Geometry: final body of the model. Coordinates: model frame, mm. A direction names the side the tool comes from. Give positions to 0.01 mm unless a question says otherwise; leave off trailing zeros. Write each loop counter-clockwise with the first axis right and the second up, starting at its lowest first coordinate (ties: lowest second). Pieces come first, ordered by that corner, then holes. Notation, with made-up numbers: (40, 41.25) -> (44, 41.25) arc R25 ccw to (44, 67.25) -> close; hole circle Ø3 at (-0.75, 44.5). An arc over 180 degrees is marked (long way). Answer as a JSON object with one key per item and string values.
from build123d import *

# Parameters (mm, degrees)
F1_DEPTH = 25


with BuildPart() as f1:
    # F0 (on Top) → F1 (new body)
    with BuildSketch(Plane.XY):
        with BuildLine():
            ThreePointArc((-17.217742, 262.83602), (-229.349777, 174.968054), (-317.217742, -37.16398))
            Line((-317.217742, -37.16398), (-287.217742, -37.16398))
            ThreePointArc((-287.217742, -37.16398), (-286.799458, -22.140706), (-285.5459, -7.16398))
            ThreePointArc((-285.5459, -7.16398), (-256.973949, 87.001077), (-196.554829, 164.673106))
            ThreePointArc((-196.554829, 164.673106), (-190.879041, 169.576808), (-185.069229, 174.320956))
            ThreePointArc((-185.069229, 174.320956), (-109.629828, 216.52876), (-24.717742, 232.731833))
            ThreePointArc((-24.717742, 232.731833), (-17.217742, 232.83602), (-9.717742, 232.731833))
            ThreePointArc((-9.717742, 232.731833), (75.194344, 216.52876), (150.633745, 174.320956))
            ThreePointArc((150.633745, 174.320956), (156.443556, 169.576808), (162.119344, 164.673106))
            ThreePointArc((162.119344, 164.673106), (222.538464, 87.001077), (251.110415, -7.16398))
            ThreePointArc((251.110415, -7.16398), (252.363973, -22.140706), (252.782258, -37.16398))
            Line((252.782258, -37.16398), (282.782258, -37.16398))
            ThreePointArc((282.782258, -37.16398), (194.914292, 174.968054), (-17.217742, 262.83602))
        make_face()
        with BuildLine():
            ThreePointArc((-285.5459, -7.16398), (-286.799458, -22.140706), (-287.217742, -37.16398))
            Line((-287.217742, -37.16398), (252.782258, -37.16398))
            ThreePointArc((252.782258, -37.16398), (252.363973, -22.140706), (251.110415, -7.16398))
            Line((251.110415, -7.16398), (-9.717742, -7.16398))
            Line((-9.717742, -7.16398), (162.119344, 164.673106))
            ThreePointArc((162.119344, 164.673106), (156.443556, 169.576808), (150.633745, 174.320956))
            Line((150.633745, 174.320956), (-9.717742, 14.049223))
            Line((-9.717742, 14.049223), (-9.717742, 232.731833))
            ThreePointArc((-9.717742, 232.731833), (-17.217742, 232.83602), (-24.717742, 232.731833))
            Line((-24.717742, 232.731833), (-24.717742, 14.049223))
            Line((-24.717742, 14.049223), (-185.069229, 174.320956))
            ThreePointArc((-185.069229, 174.320956), (-190.879041, 169.576808), (-196.554829, 164.673106))
            Line((-196.554829, 164.673106), (-24.717742, -7.16398))
            Line((-24.717742, -7.16398), (-285.5459, -7.16398))
        make_face()
    extrude(amount=F1_DEPTH)


solid = f1.part
Q1. Cut plane D-D (x = 34.5). Return the cut outline in (y, z).
Values:
{"outline": "(-37.16, 0) -> (-7.16, 0) -> (-7.16, 25) -> (-37.16, 25) -> close; (37.05, 0) -> (58.24, 0) -> (58.24, 25) -> (37.05, 25) -> close; (227.84, 0) -> (258.34, 0) -> (258.34, 25) -> (227.84, 25) -> close"}
Q2. Set-up query: faces 1 (the flat face through (-21, 82, 25)), 2 (the flat face through (-111.84, 79.96, 12.32)). Return all of +Z, -Z, +X, -X, +Y, -Y with unobstructed straight access to the full face (end or side cutting, diameter ignored); none if empty.
Values:
{"face 1": "+Z, +X, -X, +Y, -Y", "face 2": "+Z, -Z"}
Q3. Mould query, pull axis Y, two halves, no side actions, for faces 3 (the flat face through (-21, -37.164, 12)), 4 (the flat face through (71.58, 95.307, 12.325)), 5 (the flat face through (-21, 82, 0)). Classes: pulls with the +Y half, pulls with the -Y half, needs draft (parallel to the pull), parting line crosses it, or undercut.
Values:
{"face 3": "pulls with the -Y half", "face 4": "undercut", "face 5": "needs draft"}
Q4. Cut plane C-C (x = -256.5). Return the cut outline in (y, z).
Values:
{"outline": "(-37.16, 0) -> (-7.16, 0) -> (-7.16, 25) -> (-37.16, 25) -> close; (87.91, 0) -> (143.79, 0) -> (143.79, 25) -> (87.91, 25) -> close"}
Q5. Cut plane B-B (y = 86). Return the cut outline in (x, z), and give its area (3 significant figures).
Values:
{"outline": "(-290.77, 0) -> (-257.49, 0) -> (-257.49, 25) -> (-290.77, 25) -> close; (-117.88, 0) -> (-96.7, 0) -> (-96.7, 25) -> (-117.88, 25) -> close; (-24.72, 0) -> (-9.72, 0) -> (-9.72, 25) -> (-24.72, 25) -> close; (62.27, 0) -> (83.45, 0) -> (83.45, 25) -> (62.27, 25) -> close; (223.05, 0) -> (256.33, 0) -> (256.33, 25) -> (223.05, 25) -> close", "area": "3,100 mm²"}
Q6. Material intervals for L1, parallel to Y at x = -36, z = 8; L2, parallel to Y at x = 39.5, z = 18.5; L3, parallel to X at y = 115, z = 3.5, sorted ascending. Write a range as from..to.
Values:
{"L1": "-37.16..-7.16, 4.12..25.33, 232.18..262.25", "L2": "-37.16..-7.16, 42.05..63.24, 226.81..257.43", "L3": "-275.76..-240.26, -146.88..-125.72, -24.72..-9.72, 91.28..112.45, 205.82..241.33"}
Q7. First-contact query: P1, Ø12, axis at y = 186, z = 4, coming from the -X side; P2, Ø5, axis at y = 58, z = 6.5, coming from the -X side; P3, Ø7.5, axis at x = -101, z = 13, coming from the +Y side. Flat tips, straight axial feed; report the tip coordinate or a pass-through.
Values:
{"P1": "x = -224.2", "P2": "x = -302.55", "P3": "y = 251.96"}
Q8. Cut plane A-A (z = 13.25). Return the cut outline in (x, y).
Values:
{"outline": "(-317.22, -37.16) -> (282.78, -37.16) arc R300 ccw to (-17.22, 262.84) arc R300 ccw to start; hole (-285.55, -7.16) -> (-24.72, -7.16) -> (-196.55, 164.67) arc R270 ccw to start; hole (-185.07, 174.32) -> (-24.72, 14.05) -> (-24.72, 232.73) arc R270 ccw to start; hole (-9.72, -7.16) -> (251.11, -7.16) arc R270 ccw to (162.12, 164.67) -> close; hole (-9.72, 14.05) -> (150.63, 174.32) arc R270 ccw to (-9.72, 232.73) -> close"}
